```python
from build123d import *

# Parameters (mm, degrees)
SKETCH1_R               = 16
SKETCH1_R_2             = 12.7
BOSS_EXTRUDE1_DEPTH     = 40
SKETCH2_R               = 16
BOSS_EXTRUDE2_DEPTH     = 10
SKETCH3_W               = 5
SKETCH3_H               = 20
BOSS_EXTRUDE3_DEPTH     = 20
CUT_EXTRUDE1_DEPTH      = 15
CUT_EXTRUDE1_DEPTH_BACK = 5


with BuildPart() as part:
    # Sketch1 → Boss-Extrude1 (new body)
    with BuildSketch(Plane(origin=(0, 0, 0), x_dir=(1, 0, 0), z_dir=(0, 1, 0))):
        with Locations(Location((0, 0, 0), (0, 0, 270))):
            Circle(SKETCH1_R)
        with Locations(Location((0, 0, 0), (0, 0, 270))):
            Circle(SKETCH1_R_2, mode=Mode.SUBTRACT)
    extrude(amount=BOSS_EXTRUDE1_DEPTH)

    # Sketch2 → Boss-Extrude2 (add)
    with BuildSketch(Plane(origin=(0, 40, 0), x_dir=(1, 0, 0), z_dir=(0, 1, 0))):
        with Locations(Location((0, 0, 0), (0, 0, 270))):
            Circle(SKETCH2_R)
    extrude(amount=BOSS_EXTRUDE2_DEPTH)

    # Sketch3 → Boss-Extrude3 (add)
    with BuildSketch(Plane(origin=(0, 50, 0), x_dir=(1, 0, 0), z_dir=(0, 1, 0))):
        with Locations((-5, 0)):
            Rectangle(SKETCH3_W, SKETCH3_H)
        with Locations((5, 0)):
            Rectangle(SKETCH3_W, SKETCH3_H)
    extrude(amount=BOSS_EXTRUDE3_DEPTH)

    # Sketch4 → Cut-Extrude1 (cut, two sides: drawn at the far end of the back side and taken through both)
    with BuildSketch(Plane.ZY.offset(-2.5).offset(-CUT_EXTRUDE1_DEPTH_BACK)):
        with BuildLine():
            Line((0, 70), (-10, 70))
            Line((-10, 70), (-10, 60))
            ThreePointArc((-10, 60), (-7.071067812, 67.071067812), (0, 70))
        make_face()
        with BuildLine():
            Line((10, 70), (0, 70))
            ThreePointArc((0, 70), (7.071067812, 67.071067812), (10, 60))
            Line((10, 60), (10, 70))
        make_face()
        with BuildLine():
            Line((0, 58), (0, 62))
            ThreePointArc((0, 62), (-2, 60), (0, 58))
        make_face()
        with BuildLine():
            ThreePointArc((2, 60), (1.414213562, 61.414213562), (0, 62))
            Line((0, 62), (0, 58))
            ThreePointArc((0, 58), (1.414213562, 58.585786438), (2, 60))
        make_face()
    extrude(amount=CUT_EXTRUDE1_DEPTH + CUT_EXTRUDE1_DEPTH_BACK, mode=Mode.SUBTRACT)


solid = part.part
```
Here's how the part is built. I have some questions about the finished solid (model axes, mm). A direction names the side the tool comes from. Give positions to 0.01 mm unless a question says otherwise; leave off trailing zeros. Write each loop counter-clockwise with the first axis right and the second up, starting at its lowest first coordinate (ties: lowest second). Pieces come first, ordered by that corner, then holes.
(1) Imagine slicing it at D-D, the plane z = -8. Write out the boundary of the cut face in (x, y), and give its area (3 significant figures).
Output values:
outline: (-13.86, 0) - (-9.86, 0) - (-9.86, 40) - (9.86, 40) - (9.86, 0) - (13.86, 0) - (13.86, 50) - (7.5, 50) - (7.5, 66) - (2.5, 66) - (2.5, 50) - (-2.5, 50) - (-2.5, 66) - (-7.5, 66) - (-7.5, 50) - (-13.86, 50) - close
area: 757 mm2
(2) Imagine slicing it at A-A, the plane y = 52. Write out the boundary of the cut face in (x, z), and give its area (3 significant figures).
Output values:
outline: (-7.5, -10) - (-2.5, -10) - (-2.5, 10) - (-7.5, 10) - close; (2.5, -10) - (7.5, -10) - (7.5, 10) - (2.5, 10) - close
area: 200 mm2
(3) If I drill on L1, parallel to X at y = 26, z = 0; L2, parallel to Z at x = 6, y = 50.5; L3, parallel to Y at x = 2.5, z = 12.5, over which ranges is the centre line in solid material (lowest first)?
Output values:
L1: x = -16 to -12.7, 12.7 to 16
L2: z = -10 to 10
L3: y = 0 to 50
(4) Will these pins go through, and if not, where does the flat tip stop? pin 1 (1 mm diameter, centred on x = -8.5, z = -4, fed in from +Y); pin 2 (1.5 mm diameter, centred on x = -4.5, y = 53, fed in from -Z); pin 3 (16 mm diameter, centred on y = 63.5, z = 1.5, fed in from -X).
Output values:
pin 1: stops at y = 50
pin 2: stops at z = -10
pin 3: stops at x = -7.5
(5) Imagine slicing it at C-C, the plane x = 3.5. Write out the boundary of the cut face in (y, z).
Output values:
outline: (0, -15.61) - (50, -15.61) - (50, -10) - (60, -10) arc R10 ccw to (60, 10) - (50, 10) - (50, 15.61) - (0, 15.61) - (0, 12.21) - (40, 12.21) - (40, -12.21) - (0, -12.21) - close; hole circle Ø4 at (60, 0)
(6) Imagine slicing it at B-B, the plane x = 0. Write out the boundary of the cut face in (y, z), and give its area (3 significant figures).
Output values:
outline: (0, -16) - (50, -16) - (50, 16) - (0, 16) - (0, 12.7) - (40, 12.7) - (40, -12.7) - (0, -12.7) - close
area: 584 mm2
(7) Thinking about a two-plate mould opening in X: for faces 4 (the face through (5, 55, 10)), 5 (the face through (-15.62, 24.65, -3.47)), 6 (the face through (-2.5, 57.6, 0.1)), which applies, pulls with the +X half, pulls with the -X half, needs draft (parallel to the pull), parting line crosses it, or undercut?
Output values:
face 4: needs draft
face 5: parting line crosses it
face 6: undercut
(8) On a 3-axis mill with a long thin cutter (end or side, diameter ignored), from which of +Z, -Z, +X, -X, +Y, -Y can I reach the whole of each face in a straight line? I mean faces 1 (the face through (0, 40, 0)), 2 (the face through (-5, 55, -10)), 3 (the face through (2.5, 57.6, 0.1)). Say none if no direction works.
Output values:
face 1: -Y
face 2: -Z, +X, -X, +Y
face 3: +Z, -Z, +Y
